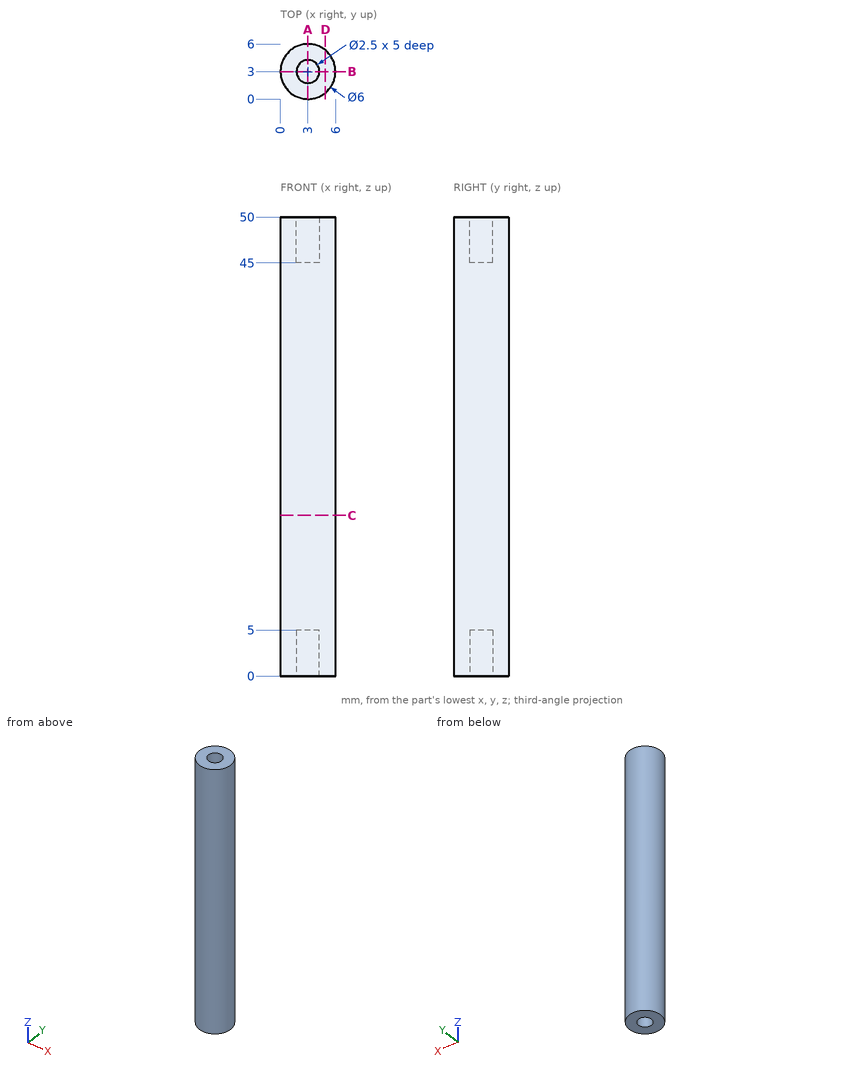
Here's the drawing with two shaded views (mm, measured from the low corner). I have some questions. Give positions to 0.01 mm unless a question says otherwise; leave off trailing zeros. Order: outer loops, then holes, each group sorted by start corner. A loop starts at its lowest first (then second) coordinate and runs counter-clockwise, first axis right, second up. Notation, with made-up numbers: (63.5, 41) -> (92.5, 41) arc R32 cw to (92.5, 70) -> close; hole circle Ø4 at (-16, 46). An arc over 180 degrees is marked (long way). Use a Markdown table: item, result. Add a question column.
Item 1: Imagine slicing it at C-C on z = 17.5. Please give me the cut outline in (x, y), plus the area to 3 significant figures.
Item 2: I need wall thicknesses on line 1 (Y direction, x = 3, z = 3.1); line 2 (Y direction, x = 3.7, z = 2); line 3 (X direction, y = 3.1, z = 21). Which ranges of each line are inside material? Lowest first, please.
Item 3: Imagine slicing it at A-A on x = 3. Please give me the cut outline in (y, z).
Item 4: Imagine slicing it at D-D on x = 4.9. Please give me the cut outline in (y, z).
Item 5: Will these pins go through, and if not, where does the flat tip stop? pin 1 (1.5 mm diameter, centred on x = 3, y = 3, fed in from +Z); pin 2 (2 mm diameter, centred on x = 3.5, y = 3, fed in from +Z); pin 3 (2 mm diameter, centred on x = 0.5, z = 20.5, fed in from +Y); pin 4 (2 mm diameter, centred on x = 5, z = 24, fed in from -Y).
Data:
| question | item | result |
|---|---|---|
| 1 | outline | circle Ø6 at (3, 3) |
| 1 | area | 28.3 mm² |
| 2 | line 1 | y = 0 to 1.75, 4.25 to 6 |
| 2 | line 2 | y = 0.08 to 1.96, 4.04 to 5.92 |
| 2 | line 3 | x = 0 to 6 |
| 3 | outline | (0, 0) -> (1.75, 0) -> (1.75, 5) -> (4.25, 5) -> (4.25, 0) -> (6, 0) -> (6, 50) -> (4.25, 50) -> (4.25, 45) -> (1.75, 45) -> (1.75, 50) -> (0, 50) -> close |
| 4 | outline | (0.68, 0) -> (5.32, 0) -> (5.32, 50) -> (0.68, 50) -> close |
| 5 | pin 1 | stops at z = 45 |
| 5 | pin 2 | stops at z = 50 |
| 5 | pin 3 | stops at y = 5.6 |
| 5 | pin 4 | stops at y = 0.17 |
